Check sheet for the drawn part. Datum: minimum x, y, z corner. Units: mm. Coordinates: 2 decimals unless noted, no trailing zeros. Order: outer loops, then holes, each group sorted by start corner. A loop starts at its lowest first (then second) coordinate and runs counter-clockwise, first axis right, second up. Notation, with made-up numbers: M 69,-13 L 113,-13 A14 cw 113,6 Z; hole C 44.25,0.25 d9. An arc over 180 degrees is marked long. Use one line per item in the form item = value. Start each with the question number.
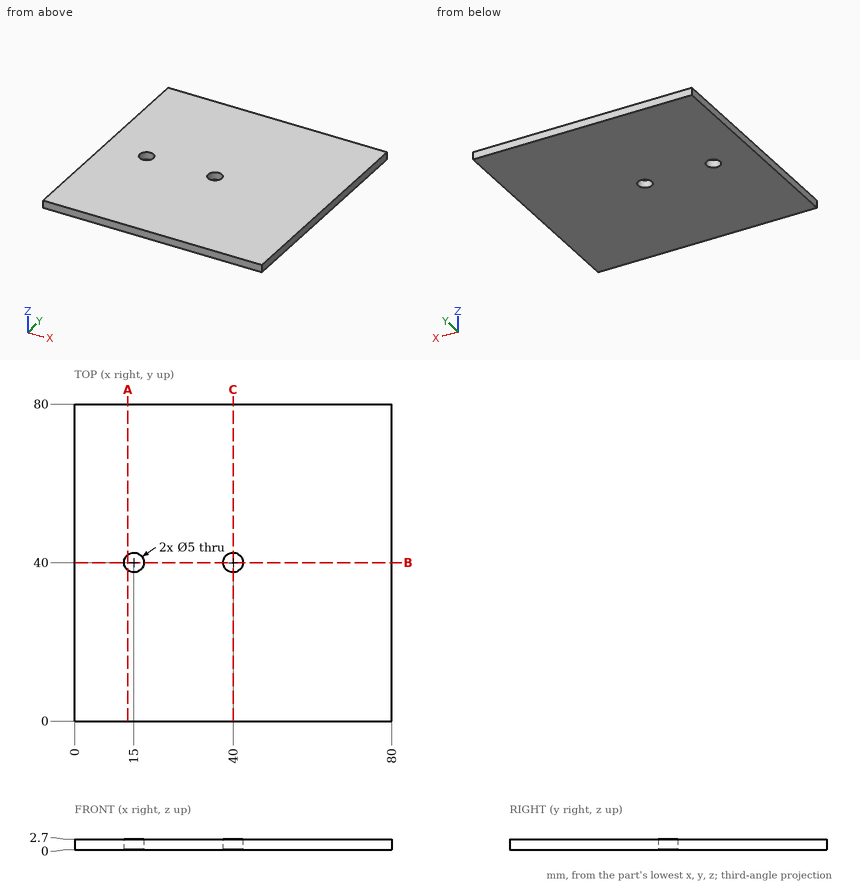
1. Cross-section at C-C on x = 40. Enter the section's corners in (y, z).
2. Cross-section at B-B on y = 40. Enter the section's corners in (x, z), and give its area (3 significant figures).
3. Material ranges on line 1 along Y through (x, z) = (40, 0.8); line 2 along X through (y, z) = (40.5, 0.2), recorded low to high.
4. Depth check by flat-ended pin: P1, Ø4, axis at x = 40, y = 40, coming from the +Z side. Enter the tip coordinate at first touch or a pass-through.
5. Cross-section at A-A on x = 13.5. Enter the section's corners in (y, z).
Final values:
q1.outline = M 0,0 L 37.5,0 L 37.5,2.7 L 0,2.7 Z; M 42.5,0 L 80,0 L 80,2.7 L 42.5,2.7 Z
q2.outline = M 0,0 L 12.5,0 L 12.5,2.7 L 0,2.7 Z; M 17.5,0 L 37.5,0 L 37.5,2.7 L 17.5,2.7 Z; M 42.5,0 L 80,0 L 80,2.7 L 42.5,2.7 Z
q2.area = 189 mm2
q3.line_1 = 0 to 37.5, 42.5 to 80
q3.line_2 = 0 to 12.55, 17.45 to 37.55, 42.45 to 80
q4.P1 = through
q5.outline = M 0,0 L 38,0 L 38,2.7 L 0,2.7 Z; M 42,0 L 80,0 L 80,2.7 L 42,2.7 Z
